Job drawing, mm, ordinate dimensions from the low corner. One solid piece. Round coordinates to 2 decimals unless told otherwise and drop trailing zeros. Write each loop counter-clockwise with the first axis right and the second up, starting at its lowest first coordinate (ties: lowest second). Pieces come first, ordered by that corner, then holes. Notation, with made-up numbers: (88.25, 38.25) -> (117.25, 38.25) arc R24 cw to (117.25, 63.25) -> close; hole circle Ø5 at (-8, -6.5). An arc over 180 degrees is marked (long way). Use CSV: the item, a comma, the result in double quotes. Start each with the question number.
(1) Saw through at A-A (y = 6). Give the cut face in (x, z), plus the area to 3 significant figures.
(2) Drop flat-ended pins along their axis: pin 1 (3 mm diameter, centred on x = 2.5, z = 16, fed in from +Y); pin 2 (2.5 mm diameter, centred on x = 5.5, y = 6, fed in from -Z); pin 3 (1.5 mm diameter, centred on y = 10.5, z = 99.5, fed in from -X); pin 4 (6 mm diameter, centred on x = 5.5, y = 6.5, fed in from +Z). Give the stop position or say it passes through.
(3) Saw through at D-D (z = 44.5). Give the cut face in (x, y).
(4) Saw through at C-C (z = 8.5). Give the cut face in (x, y).
(5) Probe line 1 (Y direction, x = 6, z = 6.5); line 2 (Z direction, x = 5.75, y = 4.5). List the from-to ranges inside material, lowest first. Write a range as [from, to].
(6) Saw through at B-B (x = 6). Give the cut face in (y, z), plus the area to 3 significant figures.
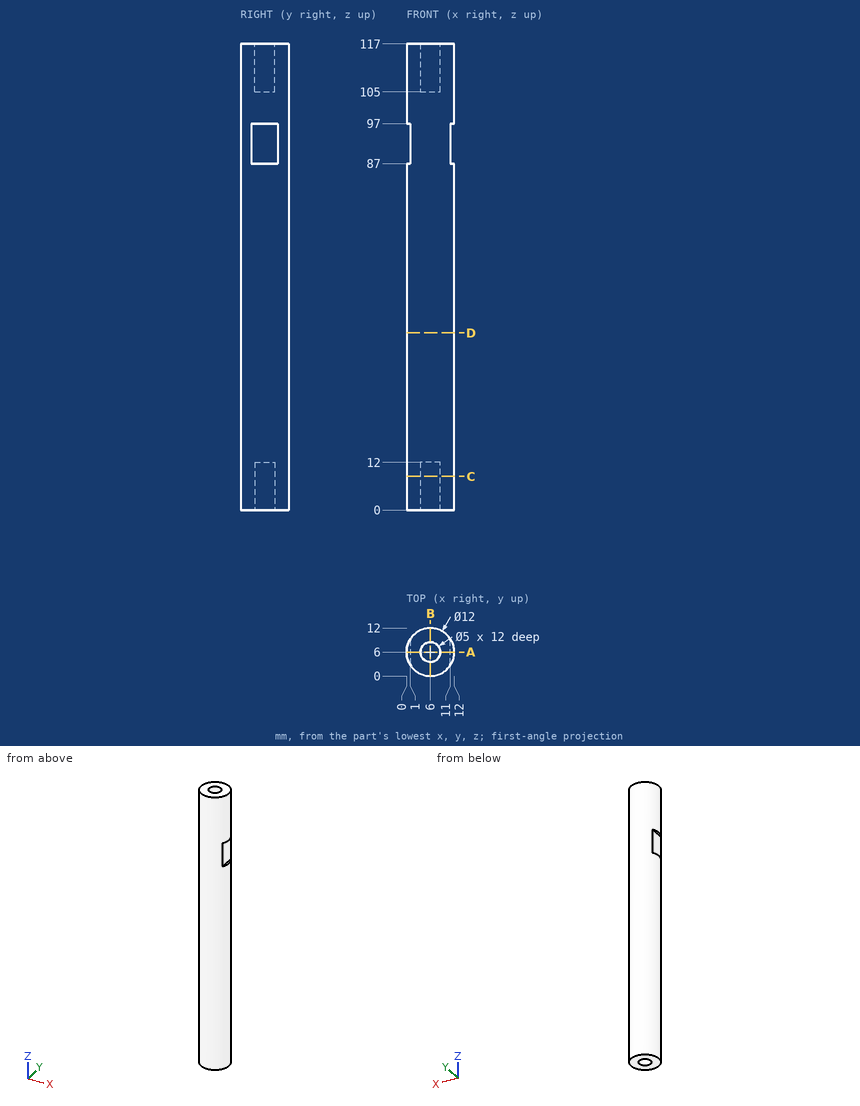
Answers:
1,outline,"(0, 0) -> (3.5, 0) -> (3.5, 12) -> (8.5, 12) -> (8.5, 0) -> (12, 0) -> (12, 87) -> (11, 87) -> (11, 97) -> (12, 97) -> (12, 117) -> (8.5, 117) -> (8.5, 105) -> (3.5, 105) -> (3.5, 117) -> (0, 117) -> (0, 97) -> (1, 97) -> (1, 87) -> (0, 87) -> close"
1,area,"1,260 mm²"
2,pin 1,"stops at y = 11.66"
2,pin 2,"stops at z = 12"
2,pin 3,"stops at x = 1.32"
2,pin 4,"stops at z = 117"
3,outline,"circle Ø12 at (6, 6)"
4,outline,"circle Ø12 at (6, 6); hole circle Ø5 at (6, 6)"
5,line 1,"y = [0, 3.5], [8.5, 12]"
5,line 2,"z = [12, 105]"
6,outline,"(0, 0) -> (3.5, 0) -> (3.5, 12) -> (8.5, 12) -> (8.5, 0) -> (12, 0) -> (12, 117) -> (8.5, 117) -> (8.5, 105) -> (3.5, 105) -> (3.5, 117) -> (0, 117) -> close"
6,area,"1,280 mm²"
